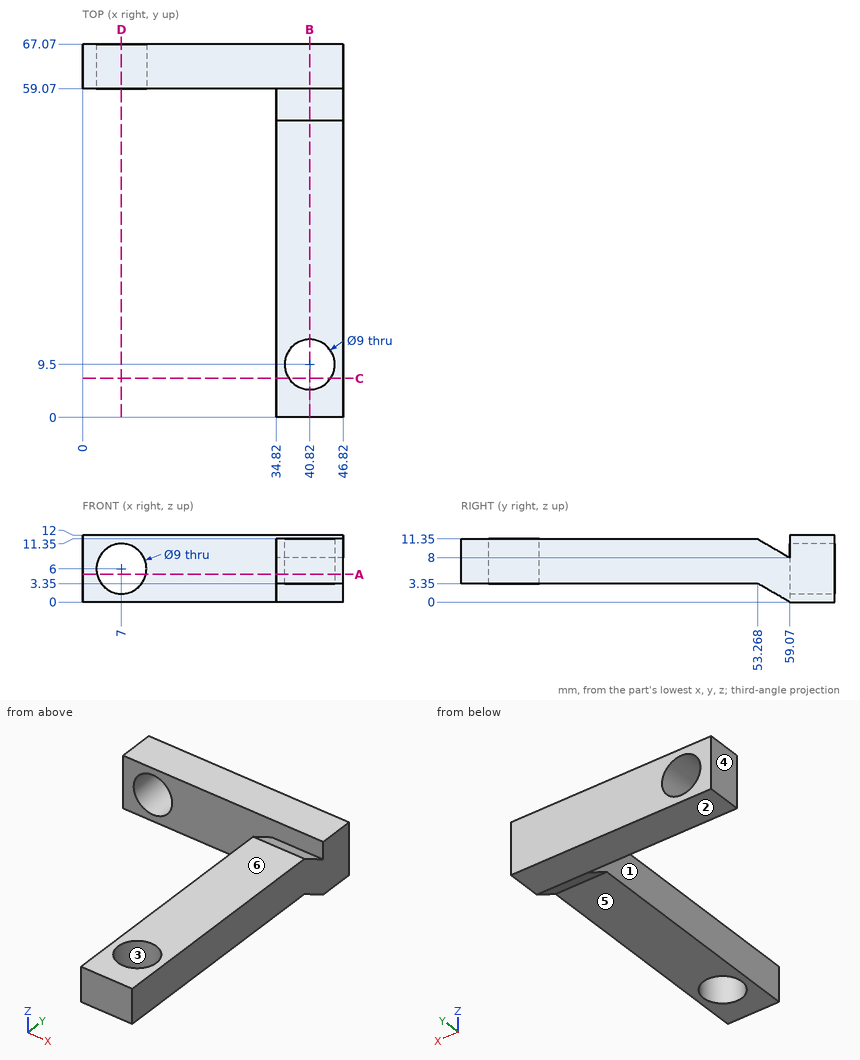
Design review of the part shown in the three views and the two pictorial views. Dimensions are in mm from the part's minimum x, y and z. A direction names the side the tool comes from. Give positions to 0.01 mm unless a question says otherwise; leave off trailing zeros. Write each loop counter-clockwise with the first axis right and the second up, starting at its lowest first coordinate (ties: lowest second). Pieces come first, ordered by that corner, then holes.
Item 1: Wall thickness on probe 1 along Y at (x, z) = (40.82, 7); probe 2 along X at (y, z) = (63, 6); probe 3 along Y at (x, z) = (41, 9.25) (1 decimal): over which ranges is each line inside the solid? List them lowest first.
Item 2: Take a section at A-A (z = 5). Give the boundary of the cut face in (x, y).
Item 3: Machinability: for the marked faces 4, 5 and 6, which of the approach directions +Z, -Z, +X, -X, +Y, -Y give a long, thin tool a straight path to every point of the face, cutting with its end or side? Answer none if there is none.
Item 4: Take a section at D-D (x = 7). Give the boundary of the cut face in (y, z), and give its area (3 significant figures).
Item 5: Insertion check: P1, Ø6, axis at x = 8, z = 4, coming from the -Y side; P2, Ø5.5, axis at x = 40.82, y = 9.5, coming from the -Z side; P3, Ø4, axis at x = 37.5, y = 46.5, coming from the +Z side; P4, Ø6, axis at x = 40, y = 24, coming from the -Z side. Each pin has a flat end and moves straight along its axis. Give the tip position at first contact, or say it passes through.
Item 6: Take a section at C-C (y = 7). Give the boundary of the cut face in (x, z).
Item 7: Take a section at B-B (x = 40.82). Give the boundary of the cut face in (y, z).
Item 8: The part is to be moulded in two halves that separate along X. For the marked faces 1, 2 and 3, say which applies: +X half, -X half, draft (parallel to the pull), parting line (faces both ways), or undercut.
Established:
1. probe 1: y = 0 to 5, 14 to 67.07
1. probe 2: x = 0 to 2.5, 11.5 to 46.82
1. probe 3: y = 0 to 5, 14 to 56.9, 59.1 to 67.1
2. outline: (0, 59.07) - (2.61, 59.07) - (2.61, 67.07) - (0, 67.07) - close; (11.39, 59.07) - (34.82, 59.07) - (34.82, 0) - (46.82, 0) - (46.82, 67.07) - (11.39, 67.07) - close; hole circle Ø9 at (40.82, 9.5)
3. face 4: +Z, -Z, -X, +Y, -Y
3. face 5: -Z, +X, -X, -Y
3. face 6: +Z, +X, -X, -Y
4. outline: (59.07, 0) - (67.07, 0) - (67.07, 1.5) - (59.07, 1.5) - close; (59.07, 10.5) - (67.07, 10.5) - (67.07, 12) - (59.07, 12) - close
4. area: 24.0 mm2
5. P1: stops at y = 59.07
5. P2: passes through
5. P3: stops at z = 11.35
5. P4: stops at z = 3.35
6. outline: (34.82, 3.35) - (37.08, 3.35) - (37.08, 11.35) - (34.82, 11.35) - close; (44.56, 3.35) - (46.82, 3.35) - (46.82, 11.35) - (44.56, 11.35) - close
7. outline: (0, 3.35) - (5, 3.35) - (5, 11.35) - (0, 11.35) - close; (14, 3.35) - (53.27, 3.35) - (59.07, 0) - (67.07, 0) - (67.07, 12) - (59.07, 12) - (59.07, 8) - (53.27, 11.35) - (14, 11.35) - close
8. face 1: -X half
8. face 2: draft
8. face 3: undercut
